```python
from build123d import *

# Parameters (mm, degrees)
SKETCH2_R           = 37.2
SKETCH2_R_2         = 15.35
BOSS_EXTRUDE1_DEPTH = 6
SKETCH3_W           = 3
SKETCH3_H           = 6
CUT_EXTRUDE1_DEPTH  = 6


with BuildPart() as part:
    # Sketch2 → Boss-Extrude1 (new body)
    with BuildSketch(Plane.XY):
        Circle(SKETCH2_R)
        Circle(SKETCH2_R_2, mode=Mode.SUBTRACT)
    extrude(amount=BOSS_EXTRUDE1_DEPTH)

    # Sketch3 → Cut-Extrude1 (cut)
    with BuildSketch(Plane.XY.offset(6)):
        with Locations((0, 34.2)):
            Rectangle(SKETCH3_W, SKETCH3_H)
        Polygon((26.269992598, -16.899038106), (31.466145021, -19.899038106), (32.966145021, -17.300961894), (27.769992598, -14.300961894), align=None)
        Polygon((-27.769992598, -14.300961894), (-32.966145021, -17.300961894), (-31.466145021, -19.899038106), (-26.269992598, -16.899038106), align=None)
    extrude(amount=-CUT_EXTRUDE1_DEPTH, mode=Mode.SUBTRACT)


solid = part.part
```
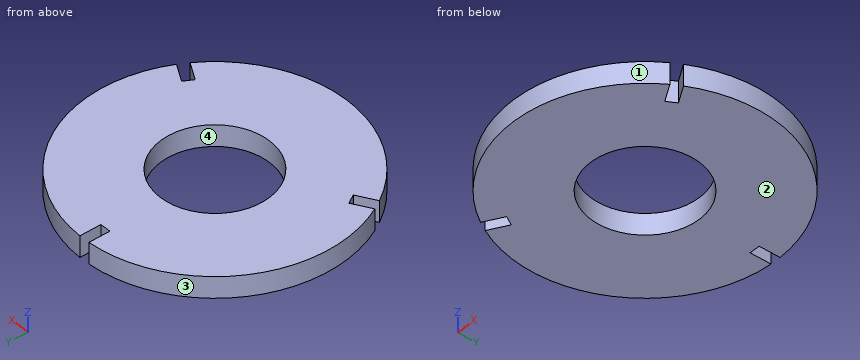
Model file for the job. Use its own axes, mm. Face numbers are marked on the shaded views. Coordinates: 2 decimals unless noted, no trailing zeros. Write each loop counter-clockwise with the first axis right and the second up, starting at its lowest first coordinate (ties: lowest second). Pieces come first, ordered by that corner, then holes. Notation, with made-up numbers: (30, -25) - (73, -25) arc R32 cw to (73, 12) - close; hole circle Ø7 at (-17, 67.5). An arc over 180 degrees is marked (long way). Use a Markdown table: item, result. Add a question column.
Item 1: Band-saw the part on C-C, the plane y = 0. Write the cut outline in (x, z), and give its area (3 significant figures).
Item 2: Two-plate mould, pull along X, no slides. Class the marked faces 1, 2, 3 and 4: pulls with the +X half, pulls with the -X half, needs draft (parallel to the pull), parting line crosses it, or undercut.
Item 3: Drop flat-ended pins along their axis: pin 1 (1.5 mm diameter, centred on x = -2.5, z = 4.5, fed in from +Y); pin 2 (6 mm diameter, centred on x = -10, y = 27, fed in from -Z); pin 3 (3 mm diameter, centred on y = 35, z = 3.5, fed in from -X); pin 4 (1 mm diameter, centred on x = -21.5, z = 4.5, fed in from -Y). Give the stop position or say it passes through.
Item 4: Band-saw the part on A-A, the plane x = 0. Write the cut outline in (y, z).
Item 5: Band-saw the part on B-B, the plane z = 1.45. Write the cut outline in (x, y), and give its area (3 significant figures).
Item 6: Drill centre lines: line 1 along Y through (x, z) = (0, 1.3); line 2 along X through (y, z) = (-0.5, 0.65); line 3 along X through (y, z) = (12.5, 4). Where is each one in solid material? Low to high.
Item 7: Band-saw the part on D-D, the plane x = -23. Write the cut outline in (y, z).
A:
| question | item | result |
|---|---|---|
| 1 | outline | (-37.2, 0) - (-15.35, 0) - (-15.35, 6) - (-37.2, 6) - close; (15.35, 0) - (37.2, 0) - (37.2, 6) - (15.35, 6) - close |
| 1 | area | 262 mm² |
| 2 | face 1 | parting line crosses it |
| 2 | face 2 | needs draft |
| 2 | face 3 | pulls with the -X half |
| 2 | face 4 | undercut |
| 3 | pin 1 | stops at y = 37.16 |
| 3 | pin 2 | stops at z = 0 |
| 3 | pin 3 | stops at x = -16.17 |
| 3 | pin 4 | stops at y = -30.71 |
| 4 | outline | (-37.2, 0) - (-15.35, 0) - (-15.35, 6) - (-37.2, 6) - close; (15.35, 0) - (31.2, 0) - (31.2, 6) - (15.35, 6) - close |
| 5 | outline | (-32.94, -17.29) - (-27.77, -14.3) - (-26.27, -16.9) - (-31.44, -19.88) arc R37.2 ccw to (31.44, -19.88) - (26.27, -16.9) - (27.77, -14.3) - (32.94, -17.29) arc R37.2 ccw to (1.5, 37.17) - (1.5, 31.2) - (-1.5, 31.2) - (-1.5, 37.17) arc R37.2 ccw to start; hole circle Ø30.7 at (0, 0) |
| 5 | area | 3,550 mm² |
| 6 | line 1 | y = -37.2 to -15.35, 15.35 to 31.2 |
| 6 | line 2 | x = -37.2 to -15.34, 15.34 to 37.2 |
| 6 | line 3 | x = -35.04 to -8.91, 8.91 to 35.04 |
| 7 | outline | (-29.24, 0) - (29.24, 0) - (29.24, 6) - (-29.24, 6) - close |
